Geometry: final body of the model. Coordinates: model frame, mm. Face numbers are marked on the shaded views. A direction names the side the tool comes from. Give positions to 0.01 mm unless a question says otherwise; leave off trailing zeros. Write each loop counter-clockwise with the first axis right and the second up, starting at its lowest first coordinate (ties: lowest second). Pieces come first, ordered by that corner, then holes.
Q1. Cut plane A-A on z = -58. Return the cut outline in (x, y).
Q2. Line query: L1, parallel to X at y = 6.25, z = 0.5; L2, parallel to X at y = 6, z = -90; L3, parallel to Z at x = 37, y = 3. Output: solid intervals per line, ascending.
Q3. Draft query along X for the marked faces 1 and 2. Return one class per face: pulls with the +X half, pulls with the -X half, needs draft (parallel to the pull), parting line crosses it, or undercut.
Q4. Cut plane B-B on x = 58. Return the cut outline in (y, z).
Q5. Cut plane D-D on y = 1.5. Count the separate pieces of the cut face and the enclosed holes in it, plus the area to 3 significant figures.
Q6. Pin query (flat end, axial travel): pin 1 (2 mm diameter, centred on x = -54, y = 5.5, fed in from +Z); pin 2 (2.5 mm diameter, centred on x = -82.71, z = -89.42, fed in from -Y); pin 3 (4.5 mm diameter, centred on x = 63.5, y = 7, fed in from -Z); pin 4 (2 mm diameter, centred on x = -18.5, y = 1, fed in from -Z). Return the tip coordinate at first contact, or that it passes through.
Q7. Cut plane C-C on x = 24. Return the cut outline in (y, z), plus the area to 3 significant figures.
Q8. Reachability of the marked faces 3 and 4 from +Z, -Z, +X, -X, +Y, -Y: full face, straight path, thin tool, end or side. Return the list, or none.
```python
from build123d import *

# Parameters (mm, degrees)
SKETCH_1_W      = 200
SKETCH_1_H      = 80
SKETCH_1_R      = 2.1
EXTRUDE_1_DEPTH = 4
SKETCH_2_W      = 200
SKETCH_2_H      = 80
SKETCH_2_W_2    = 192
SKETCH_2_H_2    = 64
SKETCH_2_R      = 6
SKETCH_2_R_2    = 2.1
EXTRUDE_4_DEPTH = 4
SKETCH_4_W      = 16
SKETCH_4_H      = 10
SKETCH_4_R      = 2.1
EXTRUDE_5_DEPTH = 8
CHAMFER_2_SIZE  = 4
CHAMFER_3_SIZE  = 2


with BuildPart() as part:
    # Эскиз1 → Бобышка-Вытянуть1 (new body)
    with BuildSketch(Plane(origin=(0, 0, 0), x_dir=(1, 0, 0), z_dir=(0, 1, 0))):
        with Locations((9.289774647, 44.419345598)):
            Rectangle(SKETCH_1_W, SKETCH_1_H)
        with Locations(Location((9.238204765, 66.885667768, 0), (0, 0, 270))):
            Circle(SKETCH_1_R, mode=Mode.SUBTRACT)
        with Locations(Location((36.096151087, 22.941432753, 0), (0, 0, 270))):
            Circle(SKETCH_1_R, mode=Mode.SUBTRACT)
        with Locations(Location((-17.619741555, 22.941432753, 0), (0, 0, 270))):
            Circle(SKETCH_1_R, mode=Mode.SUBTRACT)
        Polygon((19.089140112, 48.079252727), (27.915271652, 72.535858158), (52.411725454, 63.619878129), (43.532640104, 39.193825212), align=None, mode=Mode.SUBTRACT)
        Polygon((-33.936103706, 63.620851303), (-25.043175056, 39.187730639), (-0.611166915, 48.080254364), (-9.504095565, 72.513375028), align=None, mode=Mode.SUBTRACT)
    extrude(amount=EXTRUDE_1_DEPTH)

    # Эскиз2 → Бобышка-Вытянуть4 (add)
    # profile 1 of 5: a face of its own
    with BuildSketch(Plane(origin=(0, 4, 0), x_dir=(1, 0, 0), z_dir=(0, 1, 0))):
        with Locations((9.289774647, 44.419345598)):
            Rectangle(SKETCH_2_W, SKETCH_2_H)
        with Locations((9.289774647, 44.419345598)):
            Rectangle(SKETCH_2_W_2, SKETCH_2_H_2, mode=Mode.SUBTRACT)
    # profile 2 of 5: a face of its own
    with BuildSketch(Plane(origin=(0, 4, 0), x_dir=(1, 0, 0), z_dir=(0, 1, 0))):
        with Locations((-17.619741555, 22.941432753)):
            Circle(SKETCH_2_R)
        with Locations(Location((-17.619741555, 22.941432753, 0), (0, 0, 180))):
            Circle(SKETCH_2_R_2, mode=Mode.SUBTRACT)
    # profile 3 of 5: a face of its own
    with BuildSketch(Plane(origin=(0, 4, 0), x_dir=(1, 0, 0), z_dir=(0, 1, 0))):
        with Locations((36.096151087, 22.941432753)):
            Circle(SKETCH_2_R)
        with Locations(Location((36.096151087, 22.941432753, 0), (0, 0, 180))):
            Circle(SKETCH_2_R_2, mode=Mode.SUBTRACT)
    # profile 4 of 5: a face of its own
    with BuildSketch(Plane(origin=(0, 4, 0), x_dir=(1, 0, 0), z_dir=(0, 1, 0))):
        with BuildLine():
            Line((-23.619741555, 22.941432753), (-28.77792263, 12.419345598))
            Line((-28.77792263, 12.419345598), (47.972182779, 12.419345598))
            Line((47.972182779, 12.419345598), (42.096151087, 22.941432753))
            ThreePointArc((42.096151087, 22.941432753), (36.096151087, 16.941432753), (30.096151087, 22.941432753))
            Line((30.096151087, 22.941432753), (-11.619741555, 22.941432753))
            ThreePointArc((-11.619741555, 22.941432753), (-17.619741555, 16.941432753), (-23.619741555, 22.941432753))
        make_face()
    # profile 5 of 5: a face of its own
    with BuildSketch(Plane(origin=(0, 4, 0), x_dir=(1, 0, 0), z_dir=(0, 1, 0))):
        with BuildLine():
            Line((-25.043175056, 39.187730639), (-23.619741555, 22.941432753))
            ThreePointArc((-23.619741555, 22.941432753), (-17.619741555, 28.941432753), (-11.619741555, 22.941432753))
            Line((-11.619741555, 22.941432753), (30.096151087, 22.941432753))
            ThreePointArc((30.096151087, 22.941432753), (36.096151087, 28.941432753), (42.096151087, 22.941432753))
            Line((42.096151087, 22.941432753), (43.532640104, 39.193825212))
            Line((43.532640104, 39.193825212), (19.089140112, 48.079252727))
            Line((19.089140112, 48.079252727), (27.915271652, 72.535858158))
            Line((27.915271652, 72.535858158), (52.411725454, 63.619878129))
            Line((52.411725454, 63.619878129), (52.411725454, 76.419345598))
            Line((52.411725454, 76.419345598), (-33.936103706, 76.419345598))
            Line((-33.936103706, 76.419345598), (-33.936103706, 63.620851303))
            Line((-33.936103706, 63.620851303), (-9.504095565, 72.513375028))
            Line((-9.504095565, 72.513375028), (-0.611166915, 48.080254364))
            Line((-0.611166915, 48.080254364), (-25.043175056, 39.187730639))
        make_face()
        with Locations(Location((9.238204765, 66.885667768, 0), (0, 0, 180))):
            Circle(SKETCH_2_R_2, mode=Mode.SUBTRACT)
    extrude(amount=EXTRUDE_4_DEPTH)

    # Эскиз4 → Бобышка-Вытянуть5 (add)
    # profile 1 of 4: a face of its own
    with BuildSketch(Plane(origin=(0, 8, 0), x_dir=(1, 0, 0), z_dir=(0, 1, 0))):
        with Locations((101.289774647, 89.419345598)):
            Rectangle(SKETCH_4_W, SKETCH_4_H)
        with Locations(Location((101.289774647, 89.419345598, 0), (0, 0, 180))):
            Circle(SKETCH_4_R, mode=Mode.SUBTRACT)
    # profile 2 of 4: a face of its own
    with BuildSketch(Plane(origin=(0, 8, 0), x_dir=(1, 0, 0), z_dir=(0, 1, 0))):
        with Locations((-82.710225353, 89.419345598)):
            Rectangle(SKETCH_4_W, SKETCH_4_H)
        with Locations(Location((-82.710225353, 89.419345598, 0), (0, 0, 180))):
            Circle(SKETCH_4_R, mode=Mode.SUBTRACT)
    # profile 3 of 4: a face of its own
    with BuildSketch(Plane(origin=(0, 8, 0), x_dir=(1, 0, 0), z_dir=(0, 1, 0))):
        with Locations((101.289774647, -0.580654402)):
            Rectangle(SKETCH_4_W, SKETCH_4_H)
        with Locations(Location((101.289774647, -0.580654402, 0), (0, 0, 180))):
            Circle(SKETCH_4_R, mode=Mode.SUBTRACT)
    # profile 4 of 4: a face of its own
    with BuildSketch(Plane(origin=(0, 8, 0), x_dir=(1, 0, 0), z_dir=(0, 1, 0))):
        with Locations((-82.710225353, -0.580654402)):
            Rectangle(SKETCH_4_W, SKETCH_4_H)
        with Locations(Location((-82.710225353, -0.580654402, 0), (0, 0, 180))):
            Circle(SKETCH_4_R, mode=Mode.SUBTRACT)
    extrude(amount=-EXTRUDE_5_DEPTH)

    # Фаска2
    chamfer_2_edges = [part.edges().sort_by_distance(p)[0] for p in [
        (9.289774647, 0, -84.419345598),
        (93.289774647, 0, -89.419345598),
        (93.289774647, 0, 0.580654402),
        (-74.710225353, 0, -89.419345598),
        (9.289774647, 0, -4.419345598),
        (-74.710225353, 0, 0.580654402),
        (-90.710225353, 0, -44.419345598),
        (109.289774647, 0, -44.419345598),
    ]]
    chamfer(chamfer_2_edges, length=CHAMFER_2_SIZE)

    # Фаска3
    chamfer_3_edges = [part.edges().sort_by_distance(p)[0] for p in [
        (-33.936103706, 8, -70.020098451),
        (-12.827170986, 8, -43.633992502),
        (45.034166933, 8, -17.680389175),
        (-24.331458306, 8, -31.064581696),
        (42.814395596, 8, -31.067628982),
        (31.310890108, 8, -43.63653897),
        (40.163498553, 8, -68.077868143),
        (52.411725454, 8, -70.019611864),
        (-26.198832093, 8, -17.680389175),
        (-21.720099636, 8, -68.067113165),
    ]]
    chamfer(chamfer_3_edges, length=CHAMFER_3_SIZE)


solid = part.part
```
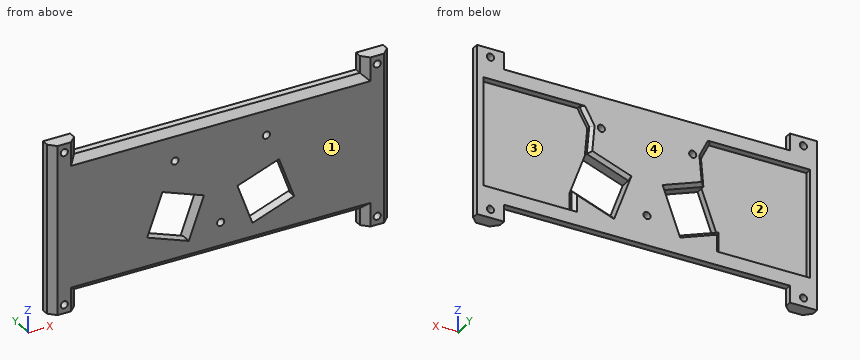
Data:
1. outline: (-90.71, 4) - (-86.71, 0) - (-31.89, 0) - (-31.89, 4) - (-86.71, 4) - (-86.71, 8) - (-90.71, 8) - close; (-4.22, 0) - (22.67, 0) - (22.67, 8) - (-4.22, 8) - close; (50.37, 0) - (105.29, 0) - (109.29, 4) - (109.29, 8) - (105.29, 8) - (105.29, 4) - (50.37, 4) - close
2. L1: x = -90.71 to -84.81, -80.61 to -74.71, 93.29 to 99.19, 103.39 to 109.29
2. L2: x = -90.71 to -84.73, -80.69 to -74.71, 93.29 to 99.27, 103.31 to 109.29
2. L3: z = -83.42 to -69.23, -41.57 to -24.84, -21.05 to -5.42
3. face 1: needs draft
3. face 2: undercut
4. outline: (0, -80.42) - (4, -84.42) - (8, -84.42) - (8, -76.42) - (4, -76.42) - (4, -12.42) - (8, -12.42) - (8, -4.42) - (4, -4.42) - (0, -8.42) - close
5. separate pieces: 1
5. enclosed holes: 9
5. area: 13,700 mm2
6. pin 1: stops at z = -4.42
6. pin 2: passes through
6. pin 3: stops at z = -84.42
6. pin 4: stops at z = -82.42
7. outline: (0, -80.42) - (4, -84.42) - (8, -84.42) - (8, -61.69) - (0, -61.69) - close; (0, -46.29) - (6, -46.29) - (8, -44.17) - (8, -4.42) - (4, -4.42) - (0, -8.42) - close
7. area: 499 mm2
8. face 3: +Y
8. face 4: +Z, -Z, +X, -X, +Y
